Solid Edge part; units mm, degrees
sketch "Sketch1" plane through (0, 0, 0) normal (0, 0, 1) x (1, 0, 0)
  line L0 (-5, -8.6603) -> (5, -8.6603)
  line L1 (5, -8.6603) -> (10, 0)
  line L2 (10, 0) -> (5, 8.6603)
  line L3 (5, 8.6603) -> (-5, 8.6603)
  line L4 (-5, 8.6603) -> (-10, 0)
  line L5 (-10, 0) -> (-5, -8.6603)
extrude "Protrusion1" add sketch "Sketch1" along normal mid plane 5
hole "Hole_1" at (0, 0, 2.5) direction (0, 0, -1) diameter 8.376 end through all
sketch "Sketch2" plane through (0, 0, 0) normal (1, 0, 0) x (0, 1, 0)
  line L0 (8.6603, -2.5) -> (27.7764, 7.0367)
revolve "RevolvedCutout1" cut sketch "Sketch2" angle 360 about axis through (0, 0, -57) along (0, 0, 1) material side at (0, 18.2407, 2.2236)
mirror "Mirror1" about plane through (0, 0, 0) normal (0, 0, 1) of "RevolvedCutout1"
properties part number "7" material "Fe 410 W"
Read the model definition and answer for the solid it produces. Units are mm, in the model's axes. Coordinates: 2 decimals unless noted, no trailing zeros. Order: outer loops, then holes, each group sorted by start corner. A loop starts at its lowest first (then second) coordinate and runs counter-clockwise, first axis right, second up. Notation, with made-up numbers: M -9,4 L 24,4 A16 cw 24,13 Z; hole C 16,28.25 d8. An arc over 180 degrees is marked long. Put each result on its own line as item: value. Start each with the question number.
Item 1: Consider probe 1 along Y at (x, z) = (0, -1.2); probe 2 along X at (y, z) = (-2, -1.5); probe 3 along X at (y, z) = (1, 0.1). Determine where each line is inside the solid, lowest interval first. Write a range as [from, to].
Item 2: The mould has two halves that part along Y. Classify faces 1 (the face through (2.83, 3.087, 0.035)), 2 (the face through (7.465, -4.391, -0.035)), 3 (the face through (-4.46, 7.8, -2.34)): +Y half, -Y half, draft (parallel to the pull), parting line (faces both ways), or undercut.
Item 3: Section A-A, the plane z = 0.25 is taken. Determine the outline of the cut face in (x, y), plus the area to 3 significant figures.
Item 4: Given pin 1 Ø3 at (y, z) = (3.5, -2) entering from -X; pin 2 Ø1 at (y, z) = (-4.5, 1) entering from -X, each flat-ended and moving along its own axis, determine where each tip first touches the part or whether it passes through.
Item 5: Section B-B, the plane z = -2.1 is taken. Determine the outline of the cut face in (x, y), plus the area to 3 significant figures.
Computed:
1. probe 1: y = [-8.66, -4.19], [4.19, 8.66]
1. probe 2: x = [-8.85, -3.68], [3.68, 8.85]
1. probe 3: x = [-9.42, -4.07], [4.07, 9.42]
2. face 1: undercut
2. face 2: -Y half
2. face 3: +Y half
3. outline: M -10,0 L -5,-8.66 L 5,-8.66 L 10,0 L 5,8.66 L -5,8.66 Z; hole C 0,0 d8.38
3. area: 205 mm2
4. pin 1: stops at x = -8.85
4. pin 2: stops at x = -7.69
5. outline: M -9.41,-1.03 L -5.59,-7.63 A9.46 ccw -3.81,-8.66 L 3.81,-8.66 A9.46 ccw 5.59,-7.63 L 9.41,-1.03 A9.46 ccw 9.41,1.03 L 5.59,7.63 A9.46 ccw 3.81,8.66 L -3.81,8.66 A9.46 ccw -5.59,7.63 L -9.41,1.03 A9.46 ccw Z; hole C 0,0 d8.38
5. area: 202 mm2
